The listing builds one solid part. Answer for the finished solid, in the listing's coordinates (mm). Face numbers are marked on the shaded views. A direction names the side the tool comes from. Give positions to 0.01 mm unless a question says otherwise; leave off trailing zeros. Loops run counter-clockwise (first coordinate to the right, second up) from the corner with the lowest first, then second, coordinate; pieces in that order, holes last. Notation, with made-up numbers: M 56.25,-24.75 L 65.25,-24.75 A33 ccw 65.25,5.25 Z; hole C 40.25,54 d4. An arc over 180 degrees is marked long. Return JSON: item names as keys, results as strings.
from build123d import *

# Parameters (mm, degrees)
BOSS_CONFIGDOWN_DEPTH = 9.525


with BuildPart() as part:
    # Sketch-ConfigDown → Boss-ConfigDown (new body)
    with BuildSketch(Plane.XY):
        with BuildLine():
            Line((6.361253842, 10.24597905), (8.738243229, 6.241984987))
            Line((8.738243229, 6.241984987), (8.057962434, 3.756033667))
            Line((8.057962434, 3.756033667), (-4.618320702, 13.379362796))
            ThreePointArc((-4.618320702, 13.379362796), (-4.527893169, 13.847264701), (-4.540792454, 14.323649986))
            ThreePointArc((-4.540792454, 14.323649986), (-5.103991925, 14.751208585), (-5.531550525, 14.188009115))
            ThreePointArc((-5.531550525, 14.188009115), (-6.110534003, 12.998511063), (-7.431054292, 13.078220852))
            ThreePointArc((-7.431054292, 13.078220852), (-8.131626042, 12.982308272), (-8.035713463, 12.281736522))
            ThreePointArc((-8.035713463, 12.281736522), (-6.795814255, 11.837551908), (-5.525309458, 12.184636302))
            Line((-5.525309458, 12.184636302), (7.950964943, 1.953985676))
            Line((7.950964943, 1.953985676), (9.277127849, 2.660583625))
            ThreePointArc((9.277127849, 2.660583625), (9.760085504, 3.061509958), (10.085312529, 2.524651128))
            ThreePointArc((10.085312529, 2.524651128), (9.565582424, 1.905135286), (8.761497669, 1.81930425))
            Line((8.761497669, 1.81930425), (7.764223808, 1.287942936))
            ThreePointArc((7.764223808, 1.287942936), (7.233567574, 0.688933561), (6.440408949, 0.582596058))
            Line((6.440408949, 0.582596058), (4.733705966, -0.326758911))
            Line((4.733705966, -0.326758911), (-6.711147083, -0.326758911))
            Line((-6.711147083, -0.326758911), (-6.711147083, -6.676758911))
            Line((-6.711147083, -6.676758911), (4.733705966, -6.676758911))
            Line((4.733705966, -6.676758911), (15.912367826, -6.676758911))
            Line((15.912367826, -6.676758911), (15.912367826, 0.083144011))
            Line((15.912367826, 0.083144011), (15.460918062, 0.556695121))
            ThreePointArc((15.460918062, 0.556695121), (14.76245819, 0.927037945), (14.425895986, 1.642388127))
            Line((14.425895986, 1.642388127), (11.670504731, 4.532673357))
            ThreePointArc((11.670504731, 4.532673357), (10.972044859, 4.903016181), (10.635482655, 5.618366363))
            Line((10.635482655, 5.618366363), (10.581235342, 6.075921255))
            Line((10.581235342, 6.075921255), (7.651089987, 11.011696177))
            ThreePointArc((7.651089987, 11.011696177), (6.623313351, 11.273755686), (6.361253842, 10.24597905))
        make_face()
        with BuildLine():
            Line((9.466844547, 0.495489391), (8.469570686, -0.035871924))
            ThreePointArc((8.469570686, -0.035871924), (7.676412061, -0.142209427), (7.145755827, -0.741218802))
            ThreePointArc((7.145755827, -0.741218802), (8.464824154, -2.274501403), (9.009980984, -0.326758911))
            Line((9.009980984, -0.326758911), (12.125210012, -0.326758911))
            ThreePointArc((12.125210012, -0.326758911), (13.158910635, -1.75798627), (14.375225055, -0.478326954))
            ThreePointArc((14.375225055, -0.478326954), (14.038662852, 0.237023228), (13.34020298, 0.607366052))
            Line((13.34020298, 0.607366052), (10.584811724, 3.497651281))
            ThreePointArc((10.584811724, 3.497651281), (10.248249521, 4.213001464), (9.549789649, 4.583344288))
            ThreePointArc((9.549789649, 4.583344288), (9.181503481, 4.313482225), (9.460673669, 3.952200837))
            Line((9.460673669, 3.952200837), (10.970207057, 2.368766163))
            Line((10.970207057, 2.368766163), (11.140648168, 2.189980874))
            ThreePointArc((11.140648168, 2.189980874), (11.42991126, 1.531140478), (10.790659406, 1.200836268))
            ThreePointArc((10.790659406, 1.200836268), (9.986574651, 1.115005233), (9.466844547, 0.495489391))
        make_face(mode=Mode.SUBTRACT)
    extrude(amount=BOSS_CONFIGDOWN_DEPTH)


solid = part.part
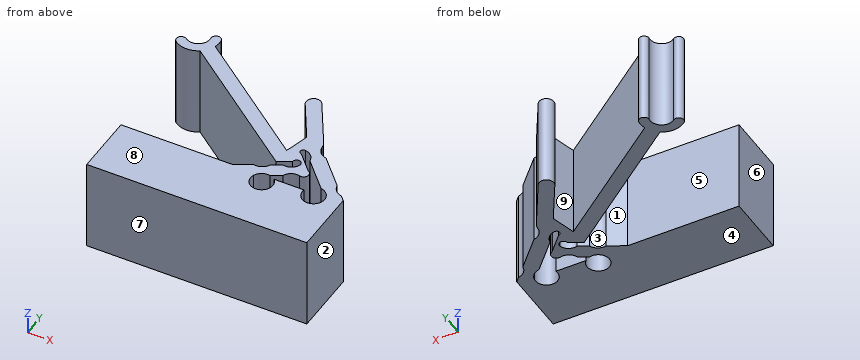
(1) The part is cut by section C-C (y = -3). Determine the outline of the cut face in (x, z) (3 decimals).
Values follow:
{"outline": "M -6.711,0 L 15.912,0 L 15.912,9.525 L -6.711,9.525 Z"}
(2) The part is cut by section A-A (x = -0.25). Determine the outline of the cut face in (y, z) (3 decimals).
Values follow:
{"outline": "M -6.677,0 L -0.327,0 L -0.327,9.525 L -6.677,9.525 Z; M 8.18,0 L 10.063,0 L 10.063,9.525 L 8.18,9.525 Z"}
(3) Straight lines are drawn through the part: line 1 along X through (y, z) = (2.25, 3.5); line 2 along X through (y, z) = (4, 3.5); line 3 along X through (y, z) = (7, 9.25). For each, find the intervals that lie inside material, in ascending order.
Values follow:
{"line 1": "7.56 to 8.51, 9.95 to 11.08, 11.77 to 13.85", "line 2": "5.26 to 7.74, 8.12 to 9.33, 10.41 to 12.18", "line 3": "1.3 to 3.78, 8.29 to 10.03"}
(4) Determine the mould class of the marked faces 1, 2, 3 and 4 for opening direction X: released by +X, released by -X, zero draft, split by the parting line, or undercut.
Values follow:
{"face 1": "released by -X", "face 2": "released by +X", "face 3": "undercut", "face 4": "zero draft"}
(5) A tool of negligible diameter and unlimited length cuts with its end or side. For the marked faces 5, 6, 7, 8 and 9, from which of +Z, -Z, +X, -X, +Y, -Y can it reach the whole face along a straight path? Write none if from no direction.
Values follow:
{"face 5": "+Z, -Z, -X", "face 6": "+Z, -Z, -X, -Y", "face 7": "+Z, -Z, +X, -X, -Y", "face 8": "+Z, +X, -X, +Y, -Y", "face 9": "+Z, -Z"}
(6) The part is cut by section B-B (y = 7). Determine the outline of the cut face in (x, z) (3 decimals), and give its area (3 significant figures).
Values follow:
{"outline": "M 1.304,0 L 3.785,0 L 3.785,9.525 L 1.304,9.525 Z; M 8.288,0 L 10.033,0 L 10.033,9.525 L 8.288,9.525 Z", "area": "40.2 mm²"}
(7) Given pin 1 (3.5 mm diameter, centred on x = 10.5, z = 2.5, fed in from +Y); pin 2 (12 mm diameter, centred on x = 7, y = -1, fed in from -Z); pin 3 (3 mm diameter, centred on y = -2, z = 4, fed in from -X); pin 4 (2 mm diameter, centred on x = 13.24, y = -0.61, fed in from +Z), each flat-ended and moving along its own axis, determine where each tip first touches the part or whether it passes through.
Values follow:
{"pin 1": "y = 9.16", "pin 2": "z = 0", "pin 3": "x = -6.71", "pin 4": "through"}
